Autodesk Inventor part; units mm, degrees
ref_plane "YZ Plane" through (0, 0, 0) normal (1, 0, 0) x (0, 1, 0)
ref_plane "XZ Plane" through (0, 0, 0) normal (0, 1, 0) x (-1, 0, 0)
ref_plane "XY Plane" through (0, 0, 0) normal (0, 0, 1) x (1, 0, 0)
sketch "Sketch1" plane through (0, 0, 0) normal (0, 1, 0) x (-1, 0, 0)
  line L0 (0, 0) -> (-160, 0)
  line L1 (-160, 0) -> (-160, 60)
  line L2 (-160, 60) -> (0, 60)
  line L3 (0, 60) -> (0, 0)
  dimension "d0" = 160
  dimension "d1" = 60
extrude "Extrusion1" add sketch "Sketch1" along normal blind 80
sketch "Sketch2" plane through (0, 80, 0) normal (0, 1, 0) x (1, 0, 0)
  line L0 (160, 0) -> (0, 0)
  line L1 (160, 0) -> (150, 0)
  line L2 (150, 0) -> (150, -10)
  line L3 (150, -10) -> (160, -10)
  line L4 (160, -10) -> (160, 0)
  line L5 (160, -10) -> (0, -10)
  line L6 (0, -10) -> (0, -40)
  line L7 (0, -40) -> (160, -40)
  line L8 (160, -40) -> (160, -10)
  dimension "d4" = 10
  dimension "d5" = 10
  dimension "d6" = 160
  dimension "d7" = 30
extrude "Extrusion2" cut sketch "Sketch2" against normal blind 70 contours L8 L7 L6 L5 L3
sketch "Sketch3" plane through (0, 80, 0) normal (0, 1, 0) x (1, 0, 0)
  line L0 (160, -40) -> (0, -40)
  line L1 (0, -40) -> (160, -40)
  line L2 (160, -40) -> (160, -50)
  line L3 (160, -50) -> (0, -50)
  line L4 (0, -50) -> (0, -40)
  point P0 (0, 0)
  dimension "d10" = 160
  dimension "d11" = 10
extrude "Extrusion3" cut sketch "Sketch3" against normal blind 10
sketch "Sketch4" plane through (160, 10, 40) normal (0, 0, -1) x (-1, 0, 0)
  line L0 (0, 0) -> (160, 0)
  arc A0 (160, 0) -> (0, 0) centre (80, -23.3333) ccw
  line L1 (0, 0) -> (0, 60)
  line L2 (0, 0) -> (0, 60)
  line L3 (0, 60) -> (80, 60)
  line L4 (160, 60) -> (0, 60)
  line L5 (160, 60) -> (160, 0)
  line L6 (160, 0) -> (160, 60)
  line L7 (160, 60) -> (80, 60)
  point P0 (160, -10)
extrude "Extrusion4" cut sketch "Sketch4" against normal blind 10 contours L1 L3 A0 | A0 L4 L5
sketch "Sketch5" plane through (160, 0, 0) normal (0, 0, -1) x (-1, 0, 0)
  line L0 (0, 80) -> (160, 80)
  line L1 (0, 80) -> (20, 80)
  line L2 (20, 80) -> (20, 30)
  line L3 (20, 30) -> (0, 30)
  line L4 (0, 30) -> (0, 80)
  line L5 (160, 10) -> (160, 80)
  line L6 (160, 80) -> (140, 80)
  line L7 (140, 80) -> (140, 30)
  line L8 (140, 30) -> (160, 30)
  line L9 (160, 30) -> (160, 80)
  point P0 (160, 0)
  dimension "d16" = 20
  dimension "d17" = 50
  dimension "d18" = 20
  dimension "d19" = 50
extrude "Extrusion5" cut sketch "Sketch5" against normal blind 10
sketch "Sketch6" plane through (0, 80, 0) normal (0, 1, 0) x (1, 0, 0)
  line L0 (20, 0) -> (20, -10)
  line L1 (20, -10) -> (140, -10)
  line L2 (140, -10) -> (140, 0)
  line L3 (140, 0) -> (20, 0)
  line L4 (20, 0) -> (20, -10)
  point P0 (0, 0)
  dimension "d22" = 120
  dimension "d23" = 10
extrude "Extrusion6" cut sketch "Sketch6" against normal blind 10
sketch "Sketch7" plane through (160, 80, 50) normal (0, 0, -1) x (-1, 0, 0)
  line L0 (0, 0) -> (0, -20)
  line L1 (0, -70) -> (0, 0)
  line L2 (0, -20) -> (0, 0)
  line L3 (160, 0) -> (0, 0)
  line L4 (0, 0) -> (60, 0)
  line L5 (60, 0) -> (0, -20)
  line L6 (0, 0) -> (160, 0)
  line L7 (160, 0) -> (160, -20)
  line L8 (160, 0) -> (160, -70)
  line L9 (160, 0) -> (100, 0)
  line L10 (100, 0) -> (160, -20)
  point P0 (160, -80)
  dimension "d26" = 20
  dimension "d27" = 60
  dimension "d28" = 20
  dimension "d29" = 60
extrude "Extrusion7" cut sketch "Sketch7" against normal blind 10
sketch "Sketch8" plane through (140, 30, 10) normal (1, 0, 0) x (0, 0, -1)
  line L0 (10, 40) -> (0, 40)
  line L1 (10, 0) -> (10, 40)
  line L2 (0, 40) -> (10, 40)
  line L3 (10, 40) -> (10, 0)
  line L4 (10, 0) -> (0, 0)
  line L5 (0, 0) -> (0, 40)
  point P0 (10, -30)
extrude "Extrusion8" cut sketch "Sketch8" against normal blind 0.5
sketch "Sketch9" plane through (20, 30, 0) normal (-1, 0, 0) x (0, 0, 1)
  line L0 (10, 40) -> (10, 0)
  line L1 (0, 0) -> (10, 0)
  line L2 (10, 40) -> (0, 40)
  line L3 (0, 40) -> (0, 0)
  line L4 (0, 0) -> (10, 0)
  line L5 (10, 0) -> (10, 40)
  point P0 (0, -30)
extrude "Extrusion9" cut sketch "Sketch9" against normal blind 0.5
sketch "Sketch11" plane through (80, -13.3333, 40) normal (0, 0, -1) x (-1, 0, 0)
  line L0 (-80, 23.3333) -> (-80, 73.3333)
  arc A0 (80, 23.3333) -> (-80, 23.3333) centre (0, 0) ccw
  line L1 (-80, 23.3333) -> (80, 23.3333)
  line L2 (-80, 23.3333) -> (80, 23.3333)
  point P0 (80, 13.3333)
extrude "Extrusion10" cut sketch "Sketch11" against normal blind 10
sketch "Sketch12" plane through (160, 10, 50) normal (0, 0, -1) x (-1, 0, 0)
  line L0 (60, 70) -> (0, 50)
  line L1 (0, 0) -> (0, 50)
  line L2 (160, 0) -> (0, 0)
  line L3 (160, 50) -> (160, 0)
  line L4 (160, 50) -> (100, 70)
  line L5 (60, 70) -> (100, 70)
  point P0 (160, -10)
extrude "Extrusion11" cut sketch "Sketch12" against normal blind 5
sketch "Sketch13" plane through (0, 10, 0) normal (0, 1, 0) x (1, 0, 0)
  line L0 (0, -55) -> (160, -55)
  line L1 (160, -55) -> (160, -40)
  line L2 (160, -40) -> (0, -40)
  line L3 (0, -40) -> (0, -55)
  point P0 (0, 0)
  dimension "d40" = 160
  dimension "d41" = 15
extrude "Extrusion12" add sketch "Sketch13" along normal blind 20
sketch "Sketch14" plane through (0, 30, 0) normal (0, 1, 0) x (1, 0, 0)
  line L0 (0, -40) -> (160, -40)
  line L1 (160, -40) -> (100, -40)
  line L2 (100, -40) -> (100, -55)
  line L3 (100, -55) -> (160, -55)
  line L4 (160, -55) -> (160, -40)
  line L5 (0, -40) -> (0, -55)
  line L6 (60, -55) -> (0, -55)
  line L7 (0, -40) -> (60, -40)
  line L8 (60, -40) -> (60, -55)
  line L9 (60, -55) -> (0, -55)
  line L10 (0, -55) -> (0, -40)
  line L11 (100, -40) -> (60, -40)
  line L12 (60, -40) -> (60, -55)
  line L13 (60, -55) -> (100, -55)
  line L14 (100, -55) -> (100, -40)
  point P0 (0, 0)
  dimension "d44" = 60
  dimension "d45" = 15
  dimension "d46" = 60
  dimension "d47" = 15
extrude "Extrusion13" cut sketch "Sketch14" against normal blind 20 contours L0 L2 L13 L8
sketch "Sketch15" plane through (0, 0, 0) normal (-1, 0, 0) x (0, 0, 1)
  line L0 (40, 30) -> (55, 30)
  line L1 (60, 0) -> (0, 0)
  line L2 (40, 30) -> (60, 30)
  line L3 (60, 30) -> (60, 0)
  line L4 (60, 0) -> (40, 0)
  line L5 (40, 0) -> (40, 30)
  line L6 (55, 80) -> (55, 60)
  line L7 (55, 60) -> (60, 60)
  line L8 (60, 60) -> (60, 30)
  line L9 (60, 30) -> (55, 30)
  line L10 (55, 30) -> (55, 60)
extrude "Extrusion14" add sketch "Sketch15" along normal blind 10
sketch "Sketch16" plane through (160, 0, 60) normal (1, 0, 0) x (0, 0, -1)
  line L0 (5, 30) -> (5, 60)
  line L1 (0, 0) -> (0, 60)
  line L2 (5, 60) -> (0, 60)
  line L3 (0, 60) -> (0, 0)
  line L4 (0, 0) -> (5, 0)
  line L5 (5, 0) -> (5, 60)
  point P0 (60, 0)
extrude "Extrusion15" add sketch "Sketch16" along normal blind 10
sketch "Sketch17" plane through (-10, 0, 0) normal (-1, 0, 0) x (0, 0, 1)
  line L0 (55, 30) -> (40, 30)
  line L1 (55, 0) -> (55, 60)
  line L2 (40, 30) -> (55, 30)
  line L3 (55, 30) -> (55, 0)
  line L4 (55, 0) -> (40, 0)
  line L5 (40, 0) -> (40, 30)
  point P0 (0, 0)
extrude "Extrusion16" cut sketch "Sketch17" against normal blind 10
sketch "Sketch18" plane through (60, 80, 60) normal (0, 0, 1) x (1, 0, 0)
  line L0 (100, -20) -> (40, 0)
  line L1 (0, 0) -> (40, 0)
  line L2 (0, 0) -> (-60, -20)
  line L3 (-60, -20) -> (-70, -20)
  line L4 (-70, -80) -> (-70, -20)
  line L5 (110, -80) -> (-70, -80)
  line L6 (110, -20) -> (110, -80)
  line L7 (100, -20) -> (110, -20)
  point P0 (-60, -80)
extrude "Extrusion17" add sketch "Sketch18" along normal blind 5
sketch "Sketch19" plane through (160, 0, 0) normal (0, 0, -1) x (-1, 0, 0)
  line L0 (0, 0) -> (60, 0)
  line L1 (160, 0) -> (0, 0)
  line L2 (60, 0) -> (100, 0)
  line L3 (100, 0) -> (100, 20)
  line L4 (100, 20) -> (60, 20)
  line L5 (60, 20) -> (60, 0)
  dimension "d58" = 60
  dimension "d59" = 40
  dimension "d60" = 20
extrude "Extrusion18" cut sketch "Sketch19" against normal blind 20
sketch "Sketch20" plane through (0, 10, 0) normal (0, 1, 0) x (1, 0, 0)
  line L0 (60, 0) -> (60, -20)
  line L1 (100, -40) -> (100, -55)
  line L2 (60, -20) -> (100, -20)
  line L3 (100, -20) -> (100, -55)
  line L4 (100, -55) -> (60, -55)
  line L5 (60, -55) -> (60, -20)
  point P0 (0, 0)
extrude "Extrusion19" cut sketch "Sketch20" against normal blind 5
sketch "Sketch21" plane through (0, 30, 0) normal (0, 1, 0) x (1, 0, 0)
  line L0 (0, -55) -> (0, 0)
  line L1 (0, -55) -> (60, -55)
  line L2 (60, -55) -> (60, -40)
  line L3 (60, -40) -> (0, -40)
  line L4 (0, -40) -> (0, -55)
  line L5 (100, -40) -> (100, -55)
  line L6 (160, -55) -> (100, -55)
  line L7 (100, -40) -> (160, -40)
  line L8 (160, -40) -> (160, -55)
  line L9 (160, -55) -> (100, -55)
  line L10 (100, -55) -> (100, -40)
extrude "Extrusion20" add sketch "Sketch21" along normal blind 10
sketch "Sketch22" plane through (160, 10, 55) normal (0, 0, -1) x (-1, 0, 0)
  line L0 (0, 50) -> (60, 70)
  line L1 (0, -10) -> (-10, -10)
  line L2 (0, 50) -> (-10, 50)
  line L3 (-10, 50) -> (-10, -10)
  line L4 (-10, -10) -> (0, -10)
  line L5 (0, -10) -> (0, 50)
  line L6 (160, 50) -> (170, 50)
  line L7 (160, -10) -> (170, -10)
  line L8 (170, -10) -> (170, 50)
  line L9 (170, 50) -> (160, 50)
  line L10 (160, 50) -> (160, -10)
extrude "Extrusion21" add sketch "Sketch22" along normal blind 15
sketch "Sketch23" plane through (0, 40, 0) normal (0, 1, 0) x (1, 0, 0)
  line L0 (160, -55) -> (160, -40)
  line L1 (100, -40) -> (160, -40)
  line L2 (160, -55) -> (100, -55)
  line L3 (100, -55) -> (100, -40)
  line L4 (100, -40) -> (160, -40)
  line L5 (160, -40) -> (160, -55)
  line L6 (0, -40) -> (60, -40)
  line L7 (60, -55) -> (0, -55)
  line L8 (60, -40) -> (0, -40)
  line L9 (0, -40) -> (0, -55)
  line L10 (0, -55) -> (60, -55)
  line L11 (60, -55) -> (60, -40)
  point P0 (0, 0)
extrude "Extrusion22" cut sketch "Sketch23" against normal blind 5
properties part number "NewLaptopSupport"
Input: part model. Units: mm. Frame: model coordinates. A direction names the side the tool comes from. Round coordinates to 2 decimals unless told otherwise and drop trailing zeros. Loops run counter-clockwise (first coordinate to the right, second up) from the corner with the lowest first, then second, coordinate; pieces in that order, holes last. Notation, with made-up numbers: (89, 82.25) -> (142, 82.25) arc R18 cw to (142, 115.25) -> close; hole circle Ø6 at (48.5, -10). An arc over 180 degrees is marked (long way). One line per item, written item: value.
(1) Pin query (flat end, axial travel): pin 1 (5.5 mm diameter, centred on x = 86.5, y = 3, fed in from -Z); pin 2 (3 mm diameter, centred on x = -6, z = 49, fed in from +Y); pin 3 (8 mm diameter, centred on y = 9, z = 19.5, fed in from -X); pin 4 (10.5 mm diameter, centred on y = 16, z = 24.5, fed in from +X). Return the tip coordinate at first contact, or that it passes through.
Geometry check:
pin 1: z = 20
pin 2: y = 60
pin 3: x = 0
pin 4: through
(2) Section C-C (y = 15.5). Return the cut outline in (x, z), plus the area to 3 significant figures.
Geometry check:
outline: (-10, 40) -> (60, 40) -> (60, 55) -> (100, 55) -> (100, 40) -> (170, 40) -> (170, 65) -> (-10, 65) -> close; (0, 0) -> (60, 0) -> (60, 10) -> (0, 10) -> close; (100, 0) -> (160, 0) -> (160, 10) -> (100, 10) -> close
area: 5,100 mm2
(3) Section A-A (x = 75). Return the cut outline in (y, z), plus the area to 4 significant figures.
Geometry check:
outline: (0, 20) -> (5, 20) -> (5, 55) -> (80, 55) -> (80, 65) -> (0, 65) -> close; (20, 0) -> (70, 0) -> (70, 10) -> (20, 10) -> close
area: 1,475 mm2
(4) Mould query, pull axis X, two halves, no side actions, for faces 1 (the face through (165, 60, 52)), 2 (the face through (160, 8, 16)), 3 (the face through (100, 9, 33)). Classes: pulls with the +X half, pulls with the -X half, needs draft (parallel to the pull), parting line crosses it, or undercut.
Geometry check:
face 1: needs draft
face 2: pulls with the +X half
face 3: undercut
(5) Set-up query: faces 4 (the face through (80, 20, 5)), 5 (the face through (139.5, 50, 5)), 6 (the face through (81, 40, 10)), 7 (the face through (-5, 60, 52)), 8 (the face through (160, 47, 48)). Return all of +Z, -Z, +X, -X, +Y, -Y with unobstructed straight access to the full face (end or side cutting, diameter ignored); none if empty.
Geometry check:
face 4: -Z, -Y
face 5: -Z, +X, +Y
face 6: +X, -X, +Y
face 7: +Z, -Z, -X, +Y
face 8: -Z, +Y
(6) Section D-D (z = 6). Return the cut outline in (x, y).
Geometry check:
outline: (0, 0) -> (60, 0) -> (60, 20) -> (100, 20) -> (100, 0) -> (160, 0) -> (160, 30) -> (139.5, 30) -> (139.5, 70) -> (20.5, 70) -> (20.5, 30) -> (0, 30) -> close
(7) Material intervals for line 1 (Z direction, x = 65, y = 33.5); line 2 (X direction, y = 16.5, z = 53); line 3 (Z direction, x = 7, y = 17), sorted ascending. Write a range as [from, to].
Geometry check:
line 1: [0, 10], [55, 65]
line 2: [-10, 60], [100, 170]
line 3: [0, 10], [40, 65]
(8) Section B-B (y = 62). Return the cut outline in (x, z), plus the area to 3 significant figures.
Geometry check:
outline: (6, 55) -> (154, 55) -> (154, 65) -> (6, 65) -> close; (20.5, 0) -> (139.5, 0) -> (139.5, 10) -> (20.5, 10) -> close
area: 2,670 mm2
